from build123d import *

# Parameters (mm, degrees)
FILLET2_R = 1


with BuildPart() as part:
    # Sketch1 → Revolve1 (revolve)
    with BuildSketch(Plane(origin=(0, 0, 0), x_dir=(1, 0, 0), z_dir=(0, 1, 0)), mode=Mode.PRIVATE) as revolve1_sk:
        Polygon((-41.5, 77), (-22, 77), (-22, 0), (-31, 0), (-31, 10), (-29.5, 10), (-29.5, 47), (-31, 47), (-31, 58), (-38, 58), (-38, 69), (-41.5, 69), align=None)
    revolve(revolve1_sk.sketch.rotate(Axis((0, 0, 0), (0, 0, -1)), 180), axis=Axis((0, 0, 0), (0, 0, -1)))  # turned: the seam where the file's is

    # Fillet2
    fillet2_edges = [part.edges().sort_by_distance(p)[0] for p in [
        (-41.5, 0, -77),
        (-41.5, 0, -69),
    ]]
    fillet(fillet2_edges, radius=FILLET2_R)


solid = part.part
Geometry: final body of the model. Coordinates: model frame, mm. A direction names the side the tool comes from. Give positions to 0.01 mm unless a question says otherwise; leave off trailing zeros. Loops run counter-clockwise (first coordinate to the right, second up) from the corner with the lowest first, then second, coordinate; pieces in that order, holes last. Notation, with made-up numbers: (34.5, -40) - (75.5, -40) arc R18 ccw to (75.5, -33) - close; hole circle Ø7 at (86, -40). An arc over 180 degrees is marked (long way). Answer as CSV lines item,"result". Start each with the question number.
1. Draft query along Z for faces 4 (the face through (-4.769, 21.477, -37.961)), 5 (the face through (14, 28, -58)), 6 (the face through (11.34, 27.41, -10)). Return one class per face: released by +Z, released by -Z, zero draft, split by the parting line, or undercut.
2. Ray query, L1, parallel to Z at x = -26.5, y = -16; L2, parallel to Y at x = 0, z = -42; L3, parallel to Y at x = 10.5, z = -42. Return the intervals inside material, ascending.
3. Section D-D, the plane z = -53. Return loops of the section in (x, y).
4. Reachability of faces 1 (the face through (28.14, -8.86, -28.76)), 2 (the face through (39.584, -12.465, -73.042)), 3 (the face through (-8.238, 37.096, -63.577)) from +Z, -Z, +X, -X, +Y, -Y: full face, straight path, thin tool, end or side. Return the list, or none.
5. Section A-A, the plane x = 0. Return loops of the section in (y, z), plus the area to 3 significant figures.
6. Section C-C, the plane z = -39. Return loops of the section in (x, y).
7. Pin query (flat end, axial travel): P1, Ø1, axis at x = 13, z = -61, coming from the +Y side; P2, Ø10, axis at x = 26.5, y = 26.5, coming from the +Z side; P3, Ø12, axis at y = 7.5, z = -63.5, coming from the +X side; P4, Ø23, axis at x = 4, y = 14, coming from the +Z side. Return the tip coordinate at first contact, or that it passes through.
Answers:
1,face 4,"zero draft"
1,face 5,"released by +Z"
1,face 6,"undercut"
2,L1,"z = -77 to -47, -10 to 0"
2,L2,"y = -29.5 to -22, 22 to 29.5"
2,L3,"y = -27.57 to -19.33, 19.33 to 27.57"
3,outline,"circle Ø62 at (0, 0); hole circle Ø44 at (0, 0)"
4,face 1,"none"
4,face 2,"+Z, -Z"
4,face 3,"+Z"
5,outline,"(-41.5, -76) arc R1 ccw to (-40.5, -77) - (-22, -77) - (-22, 0) - (-31, 0) - (-31, -10) - (-29.5, -10) - (-29.5, -47) - (-31, -47) - (-31, -58) - (-38, -58) - (-38, -69) - (-40.5, -69) arc R1 ccw to (-41.5, -70) - close; (22, -77) - (40.5, -77) arc R1 ccw to (41.5, -76) - (41.5, -70) arc R1 ccw to (40.5, -69) - (38, -69) - (38, -58) - (31, -58) - (31, -47) - (29.5, -47) - (29.5, -10) - (31, -10) - (31, 0) - (22, 0) - close"
5,area,"1,600 mm2"
6,outline,"circle Ø59 at (0, 0); hole circle Ø44 at (0, 0)"
7,P1,"stops at y = 35.89"
7,P2,"stops at z = -58"
7,P3,"stops at x = 40.8"
7,P4,"stops at z = 0"
